```python
from build123d import *

# Parameters (mm, degrees)
SKETCH_R        = 1.2
PAD_DEPTH       = 3
PAD001_DEPTH    = 10
FILLET_R        = 3
SKETCH002_R     = 2.5
POCKET_DEPTH    = 6
PAD002_DEPTH    = 7
SKETCH004_W     = 20
SKETCH004_H     = 4
POCKET001_DEPTH = 12
SKETCH006_R     = 1.2
POCKET002_DEPTH = 5
PAD003_DEPTH    = 6
SKETCH008_R     = 1.1
POCKET003_DEPTH = 5


with BuildPart() as part:
    # Sketch → Pad (new body)
    with BuildSketch(Plane.XY):
        Polygon((0, 12), (0, 0), (-20, 0), (-20, 12), (-15, 19.412805), (-5, 19.412805), align=None)
        with Locations((-13, 4)):
            Circle(SKETCH_R, mode=Mode.SUBTRACT)
        with Locations((-7, 4)):
            Circle(SKETCH_R, mode=Mode.SUBTRACT)
    extrude(amount=PAD_DEPTH)

    # Sketch001 (on Face10 of Pad) → Pad001 (join)
    with BuildSketch(Plane.XY.offset(3)):
        Polygon((-14.90374, 19.331674), (-5.09626, 19.331674), (-1.5, 14), (-18.5, 14), align=None)
    extrude(amount=PAD001_DEPTH)

    # Fillet
    fillet_edges = [part.edges().sort_by_distance(p)[0] for p in [
        (-3.29813, 16.665837, 13),
        (-10, 19.331674, 13),
        (-16.70187, 16.665837, 13),
    ]]
    fillet(fillet_edges, radius=FILLET_R)

    # Sketch002 (on Face12 of Pad001) → Pocket (cut)
    with BuildSketch(Plane.XZ.offset(-14)):
        with Locations((-10, 8)):
            Circle(SKETCH002_R)
    extrude(amount=-POCKET_DEPTH, mode=Mode.SUBTRACT)

    # Sketch003 (on Face19 of Pocket) → Pad002 (join)
    with BuildSketch(Plane(origin=(0, 0, 0), x_dir=(1, 0, 0), z_dir=(0, 0, -1))):
        Polygon((0, 0), (-20, 0), (-20, -12), (-15.004024, -19.406839), (-4.995976, -19.406839), (0, -12), align=None)
    extrude(amount=PAD002_DEPTH)

    # Sketch004 (on Face22 of Pad002) → Pocket001 (cut)
    with BuildSketch(Plane.XZ):
        with Locations((-10, -2)):
            Rectangle(SKETCH004_W, SKETCH004_H)
    extrude(amount=-POCKET001_DEPTH, mode=Mode.SUBTRACT)

    # Sketch006 (on Face26 of Pocket001) → Pocket002 (cut)
    with BuildSketch(Plane(origin=(0, 0, -7), x_dir=(1, 0, 0), z_dir=(0, 0, -1))):
        with Locations((-13, -4)):
            Circle(SKETCH006_R)
        with Locations((-7, -4)):
            Circle(SKETCH006_R)
    extrude(amount=-POCKET002_DEPTH, mode=Mode.SUBTRACT)

    # Sketch007 (on Face26 of Pocket002) → Pad003 (join)
    with BuildSketch(Plane(origin=(0, 0, -7), x_dir=(1, 0, 0), z_dir=(0, 0, -1))):
        Polygon((-10, -19.5), (-23, -19.5), (-23, -17.5), (-10, -17.5), (3, -17.5), (3, -19.5), align=None)
    extrude(amount=PAD003_DEPTH)

    # Sketch008 (on Face38 of Pad003) → Pocket003 (cut)
    with BuildSketch(Plane(origin=(0, 19.5, 0), x_dir=(-1, 0, 0), z_dir=(0, 1, 0))):
        with Locations((20.1, -8.6)):
            Circle(SKETCH008_R)
        with Locations((-0.1, -8.6)):
            Circle(SKETCH008_R)
    extrude(amount=-POCKET003_DEPTH, mode=Mode.SUBTRACT)


solid = part.part
```
Model file for the job. Use its own axes, mm. A direction names the side the tool comes from. Coordinates: 2 decimals unless noted, no trailing zeros. Loops run counter-clockwise (first coordinate to the right, second up) from the corner with the lowest first, then second, coordinate; pieces in that order, holes last. Notation, with made-up numbers: (22, 77.25) - (63, 77.25) arc R29 ccw to (63, 116.25) - close; hole circle Ø2 at (47, 3.5). An arc over 180 degrees is marked (long way). Answer as a JSON object with one key per item and string values. Group by question number.
(1) Cut at B-B (y = 10). Give the cut face in (x, z).
(2) Cut at D-D (z = 0.5). Give the cut face in (x, y), then the cut area to 3 significant figures.
(3) Two-plate mould, pull along Y, no slides. Class faces 4 (the face through (-11.855, 4.36, 1.479)), 5 (the face through (-8, 14, 6)), 6 (the face through (-3.32, 16.7, 6.45)): released by +Y, released by -Y, zero draft, split by the parting line, or undercut.
(4) Tool access for faces 1 (the face through (-16.727, 16.629, 6.451)), 2 (the face through (-10, 12, -2)), 3 (the face through (-10, 17.5, -10)): list every direction of +Z, -Z, +X, -X, +Y, -Y with a clear straight run to the whole face (end or side of a thin tool).
(5) Probe line 1 along X through (y, z) = (4, -6.3); line 2 along Z through (x, y) = (-1.25, 3.25); line 3 along Y through (x, z) = (-13, -5.1). List the from-to ranges inside material, lowest first.
(6) Flat gauge pins, fed straight in: pin 1 (3 mm diameter, centred on x = -11.5, z = 5.5, fed in from -Y); pin 2 (3 mm diameter, centred on x = -7, y = 4, fed in from -Z); pin 3 (4 mm diameter, centred on y = 8.5, z = -7, fed in from +X). Where does each tip first touch, or does it go through?
(7) Cut at A-A (z = 8). Give the cut face in (x, y).
Geometry says:
{
 "1": {"outline": "(-20, -7) - (0, -7) - (0, -4) - (-20, -4) - close; (-20, 0) - (0, 0) - (0, 3) - (-20, 3) - close"},
 "2": {"outline": "(-20, 0) - (0, 0) - (0, 12) - (-5, 19.41) - (-15, 19.41) - (-20, 12) - close; hole circle Ø2.4 at (-13, 4); hole circle Ø2.4 at (-7, 4)", "area": "342 mm^2"},
 "3": {"face 4": "undercut", "face 5": "released by -Y", "face 6": "released by +Y"},
 "4": {"face 1": "+Z, -X, +Y", "face 2": "+X, -X, -Y", "face 3": "-Z, +X, -X, -Y"},
 "5": {"line 1": "x = -20 to -14.2, -11.8 to -8.2, -5.8 to 0", "line 2": "z = -7 to -4, 0 to 3", "line 3": "y = 0 to 2.8, 5.2 to 19.41"},
 "6": {"pin 1": "stops at y = 14", "pin 2": "stops at z = -7", "pin 3": "stops at x = 0"},
 "7": {"outline": "(-18.5, 14) - (-12.5, 14) - (-12.5, 19.33) - (-14.9, 19.33) - close; (-7.5, 14) - (-1.5, 14) - (-5.1, 19.33) - (-7.5, 19.33) - close"}
}
